Work out the finished part from the listing and answer in its coordinate system (mm). A direction names the side the tool comes from. Coordinates: 2 decimals unless noted, no trailing zeros. Order: outer loops, then holes, each group sorted by start corner. A loop starts at its lowest first (then second) coordinate and runs counter-clockwise, first axis right, second up.
1. Flat-ended cylindrical pins translate along their axes: pin 1 Ø2 at (x, y) = (-11, 3) entering from -Z; pin 2 Ø3 at (x, y) = (-4.5, 1.5) entering from +Z; pin 3 Ø1.5 at (y, z) = (0, 3) entering from +X. Find the tip coordinate at first contact, or state that the pin passes through.
2. A tool of negligible diameter and unlimited length cuts with its end or side. For faces 4 (the conical face through (-2.2, -1.27, 5.74)), 5 (the flat face through (-1, 0.8, 0)), from which of +Z, -Z, +X, -X, +Y, -Y can it reach the whole face along a straight path? Write none if from no direction.
3. The part is cut by section B-B, the plane y = 0. Give the vertices of the cut face in (x, z).
4. The part is cut by section C-C, the plane x = -7. Give the vertices of the cut face in (y, z), then the cut area to 3 significant figures.
5. Determine the mould class of faces 1 (the cylindrical face through (-13, -3, 0)), 2 (the flat face through (0, 2, 0)), 3 (the flat face through (-3.6, -3, 1)) for opening direction X: +X half, -X half, draft (parallel to the pull), parting line (faces both ways), or undercut.
6. Find the intervals of material crossed by probe 1 along X at (y, z) = (-2.75, 3); probe 2 along Z at (x, y) = (-1.5, 1.25); probe 3 along Z at (x, y) = (-2, -2.25), in increasing order.
7. The part is cut by section A-A, the plane z = 0. Give the vertices of the cut face in (x, y).
```python
from build123d import *

# Parameters (mm, degrees)
SKETCH2_W          = 11.892854998
SKETCH2_H          = 1.6
CUT_EXTRUDE1_DEPTH = 1.4
CHAMFER1_SIZE      = 0.5


with BuildPart() as part:
    # Sketch1 → Revolve1 (revolve)
    with BuildSketch(Plane.XY):
        with BuildLine():
            Line((0, 0), (0, 4.035644698))
            ThreePointArc((0, 4.035644698), (-0.472900794, 5.251707072), (-1.643119663, 5.828795155))
            Line((-1.643119663, 5.828795155), (-3.6, 6))
            Line((-3.6, 6), (-3.6, 3))
            Line((-3.6, 3), (-23.6, 3))
            Line((-23.6, 3), (-23.6, 0))
            Line((-23.6, 0), (0, 0))
        make_face()
    revolve(axis=Axis((0, 0, 0), (-1, 0, 0)))

    # Sketch2 → Cut-Extrude1 (cut)
    with BuildSketch(Plane(origin=(0, 0, 0), x_dir=(0, 0, -1), z_dir=(1, 0, 0))):
        Rectangle(SKETCH2_W, SKETCH2_H)
    extrude(amount=-CUT_EXTRUDE1_DEPTH, mode=Mode.SUBTRACT)

    # Chamfer1
    chamfer1_edges = [part.edges().sort_by_distance(p)[0] for p in [
        (-23.6, -3, 0),
    ]]
    chamfer(chamfer1_edges, length=CHAMFER1_SIZE)


solid = part.part
```
Geometry says:
1. pin 1: stops at z = -2.24
1. pin 2: stops at z = 5.99
1. pin 3: stops at x = -1.4
2. face 4: +X
2. face 5: +Z, -Z, +X
3. outline: (-23.6, -2.5) - (-23.1, -3) - (-3.6, -3) - (-3.6, -6) - (-1.64, -5.83) arc R1.8 ccw to (-1.4, -5.79) - (-1.4, 5.79) arc R1.8 ccw to (-1.64, 5.83) - (-3.6, 6) - (-3.6, 3) - (-23.1, 3) - (-23.6, 2.5) - close
4. outline: circle Ø6 at (0, 0)
4. area: 28.3 mm2
5. face 1: draft
5. face 2: +X half
5. face 3: -X half
6. probe 1: x = -3.6 to 0
6. probe 2: z = -5.67 to 5.67
6. probe 3: z = -5.41 to 5.41
7. outline: (-23.6, -2.5) - (-23.1, -3) - (-3.6, -3) - (-3.6, -6) - (-1.64, -5.83) arc R1.8 ccw to (0, -4.04) - (0, -0.8) - (-1.4, -0.8) - (-1.4, 0.8) - (0, 0.8) - (0, 4.04) arc R1.8 ccw to (-1.64, 5.83) - (-3.6, 6) - (-3.6, 3) - (-23.1, 3) - (-23.6, 2.5) - close
